Check sheet for the drawn part. Datum: minimum x, y, z corner. Units: mm. A direction names the side the tool comes from. Round coordinates to 2 decimals unless told otherwise and drop trailing zeros. Write each loop counter-clockwise with the first axis right and the second up, starting at its lowest first coordinate (ties: lowest second). Pieces come first, ordered by that corner, then holes. Notation, with made-up numbers: M 46.5,85 L 85.5,85 A20 cw 85.5,122 Z; hole C 28,0 d5. An arc over 180 degrees is marked long. Use a Markdown table: item, result.
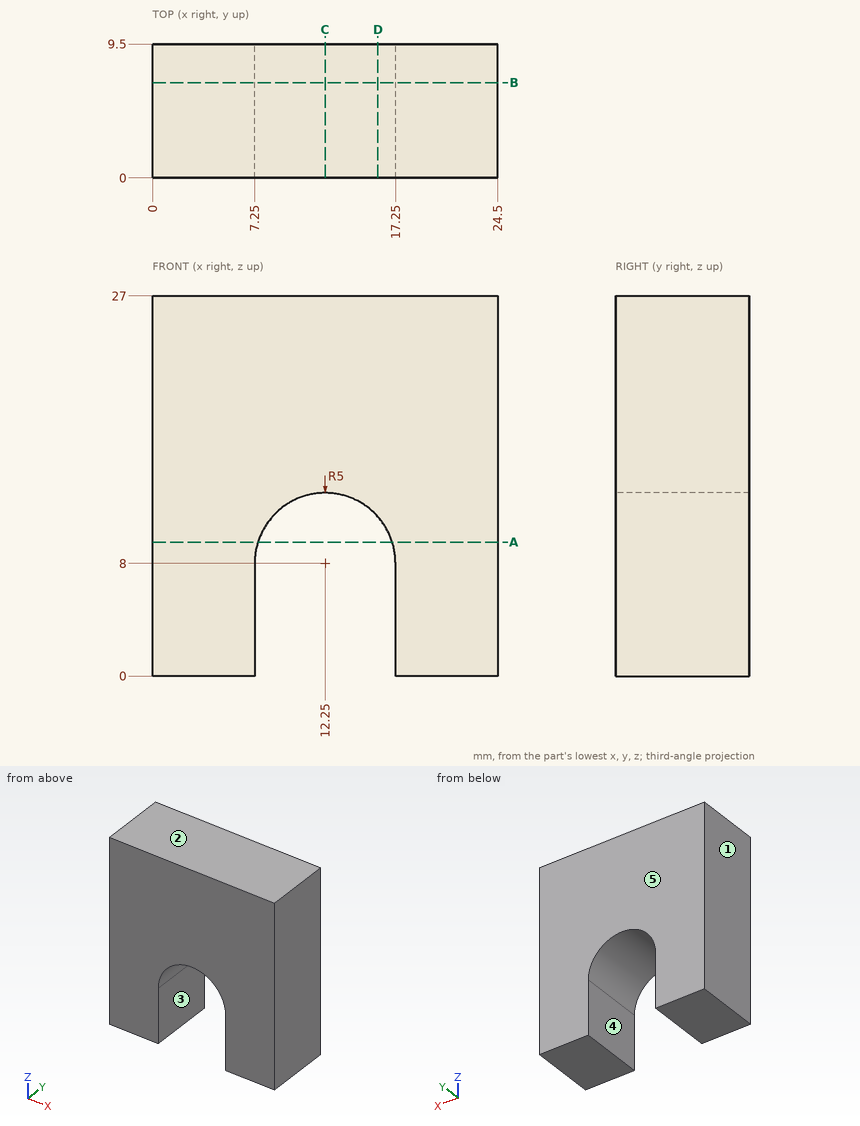
Item 1: Cross-section at D-D, the plane x = 16. Record the cut outline in (y, z).
Outcome:
| item | result |
|---|---|
| outline | M 0,11.31 L 9.5,11.31 L 9.5,27 L 0,27 Z |
Item 2: Cross-section at C-C, the plane x = 12.25. Record the cut outline in (y, z).
Outcome:
| item | result |
|---|---|
| outline | M 0,13 L 9.5,13 L 9.5,27 L 0,27 Z |
Item 3: Access from +Z, -Z, +X, -X, +Y, -Y to the whole of each face (thin tool, end or side, straight path). Record for the marked faces 4 and 5.
Outcome:
| item | result |
|---|---|
| face 4 | -Z, +Y, -Y |
| face 5 | +Z, -Z, +X, -X, +Y |
Item 4: Cross-section at B-B, the plane y = 6.75. Record the cut outline in (x, z), and give its area (3 significant figures).
Outcome:
| item | result |
|---|---|
| outline | M 0,0 L 7.25,0 L 7.25,8 A5 cw 17.25,8 L 17.25,0 L 24.5,0 L 24.5,27 L 0,27 Z |
| area | 542 mm2 |
Item 5: Cross-section at A-A, the plane z = 9.5. Record the cut outline in (x, y), and give its area (3 significant figures).
Outcome:
| item | result |
|---|---|
| outline | M 0,0 L 7.48,0 L 7.48,9.5 L 0,9.5 Z; M 17.02,0 L 24.5,0 L 24.5,9.5 L 17.02,9.5 Z |
| area | 142 mm2 |
Item 6: Go/stop test with a flat-tipped pin: pin 1 (2 mm diameter, centred on x = 12, z = 10, fed in from -Y). Record where the tip stops, or that it passes through.
Outcome:
| item | result |
|---|---|
| pin 1 | passes through |
Item 7: Mould release check, pull along X, two halves, no side actions. Record for the marked faces 1, 2 and 3: +X half, -X half, draft (parallel to the pull), parting line (faces both ways), or undercut.
Outcome:
| item | result |
|---|---|
| face 1 | -X half |
| face 2 | draft |
| face 3 | undercut |
Item 8: Material ranges on line 1 along X through (y, z) = (3.25, 8); line 2 along Z through (x, y) = (12.25, 0.5); line 3 along Z through (x, y) = (11.5, 8.75), recorded low to high. Write a range as from..to.
Outcome:
| item | result |
|---|---|
| line 1 | x = 0..7.25, 17.25..24.5 |
| line 2 | z = 13..27 |
| line 3 | z = 12.94..27 |
